Verification items for the finished model (mm, model axes). Face numbers are marked on the shaded views. A direction names the side the tool comes from. Coordinates: 2 decimals unless noted, no trailing zeros. Order: outer loops, then holes, each group sorted by start corner. A loop starts at its lowest first (then second) coordinate and runs counter-clockwise, first axis right, second up. Notation, with made-up numbers: (44, 29) -> (77, 29) arc R13 ccw to (77, 47) -> close; hole circle Ø4 at (50.25, -7). An arc over 180 degrees is marked (long way). Answer as CSV lines item,"result".
```python
from build123d import *

# Parameters (mm, degrees)
SKETCH1_W           = 19.82
SKETCH1_H           = 4.8
BOSS_EXTRUDE1_DEPTH = 3.81
SKETCH2_W           = 3.81
SKETCH2_H           = 4.8
BOSS_EXTRUDE2_DEPTH = 11.89
SKETCH3_W           = 3.81
SKETCH3_H           = 3.81
BOSS_EXTRUDE3_DEPTH = 22.5
SKETCH4_W           = 19.82
SKETCH4_H           = 3.81
BOSS_EXTRUDE4_DEPTH = 2.54


with BuildPart() as part:
    # Sketch1 → Boss-Extrude1 (new body)
    with BuildSketch(Plane(origin=(0, 0, 0), x_dir=(1, 0, 0), z_dir=(0, 1, 0))):
        with Locations((34.380252927, 12.547082461)):
            Rectangle(SKETCH1_W, SKETCH1_H)
    extrude(amount=BOSS_EXTRUDE1_DEPTH)

    # Sketch2 → Boss-Extrude2 (add)
    with BuildSketch(Plane.XZ):
        with Locations((26.375252927, -12.547082461)):
            Rectangle(SKETCH2_W, SKETCH2_H)
        with Locations((42.385252927, -12.547082461)):
            Rectangle(SKETCH2_W, SKETCH2_H)
    extrude(amount=BOSS_EXTRUDE2_DEPTH)

    # Sketch3 → Boss-Extrude3 (add)
    with BuildSketch(Plane(origin=(0, 0, -14.947082461), x_dir=(-1, 0, 0), z_dir=(0, 0, -1))):
        with Locations((-42.385252927, -9.985)):
            Rectangle(SKETCH3_W, SKETCH3_H)
        with Locations((-26.375252927, -9.985)):
            Rectangle(SKETCH3_W, SKETCH3_H)
    extrude(amount=BOSS_EXTRUDE3_DEPTH)

    # Sketch4 → Boss-Extrude4 (add)
    with BuildSketch(Plane(origin=(0, 0, -37.447082461), x_dir=(-1, 0, 0), z_dir=(0, 0, -1))):
        with Locations((-34.380252927, -9.985)):
            Rectangle(SKETCH4_W, SKETCH4_H)
    extrude(amount=BOSS_EXTRUDE4_DEPTH)


solid = part.part
```
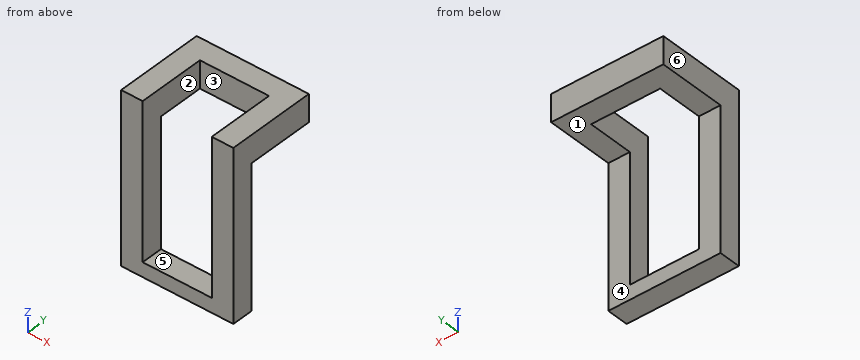
Item 1: Section check D-D, the plane y = -10.5. Record the boundary of the cut face in (x, z), plus the area to 3 significant figures.
Answer list:
outline,"(24.47, -39.99) -> (44.29, -39.99) -> (44.29, -10.15) -> (40.48, -10.15) -> (40.48, -37.45) -> (28.28, -37.45) -> (28.28, -10.15) -> (24.47, -10.15) -> close"
area,"258 mm2"
Item 2: Release check for a two-part mould opening along X. For the marked faces 4, 5 and 6 record: +X half, -X half, draft (parallel to the pull), parting line (faces both ways), or undercut.
Answer list:
face 4,"draft"
face 5,"undercut"
face 6,"-X half"
Item 3: Thickness scan on line 1 (X direction, y = -10.75, z = -35.25); line 2 (Y direction, x = 31.5, z = -12.25); line 3 (Y direction, x = 41.5, z = -31). Record the ranges inside material, lowest first.
Answer list:
line 1,"24.47 to 28.28, 40.48 to 44.29"
line 2,"0 to 3.81"
line 3,"-11.89 to -8.08"
Item 4: Depth check by flat-ended pin: pin 1 Ø6 at (x, y) = (32, -2) entering from -Z; pin 2 Ø3 at (x, y) = (34.5, -9.5) entering from +Z; pin 3 Ø2 at (x, y) = (36, -1.5) entering from +Z; pin 4 Ø5 at (x, z) = (41.5, -25.5) entering from +Y. Enter the tip coordinate at first touch or a pass-through.
Answer list:
pin 1,"z = -14.95"
pin 2,"z = -37.45"
pin 3,"through"
pin 4,"y = -8.08"
Item 5: Section check C-C, the plane x = 27.25. Record the boundary of the cut face in (y, z).
Answer list:
outline,"(-11.89, -39.99) -> (-8.08, -39.99) -> (-8.08, -14.95) -> (3.81, -14.95) -> (3.81, -10.15) -> (-11.89, -10.15) -> close"
Item 6: Tool access check on the marked faces 1, 2 and 3. Record the directions out of +Z, -Z, +X, -X, +Y, -Y that give a thin tool (end or side, any length) a straight path to the whole face; none if there is none.
Answer list:
face 1,"-Z, +X, -X, +Y"
face 2,"+Z, -Y"
face 3,"+Z, -Z, -Y"
Item 7: Section check A-A, the plane z = -26.75. Record the boundary of the cut face in (x, y).
Answer list:
outline,"(24.47, -11.89) -> (28.28, -11.89) -> (28.28, -8.08) -> (24.47, -8.08) -> close; (40.48, -11.89) -> (44.29, -11.89) -> (44.29, -8.08) -> (40.48, -8.08) -> close"
Item 8: Section check B-B, the plane y = -1.5. Record the boundary of the cut face in (x, z).
Answer list:
outline,"(24.47, -14.95) -> (28.28, -14.95) -> (28.28, -10.15) -> (24.47, -10.15) -> close; (40.48, -14.95) -> (44.29, -14.95) -> (44.29, -10.15) -> (40.48, -10.15) -> close"
